Part model, mm, in its own coordinate system. Round coordinates to 2 decimals unless told otherwise and drop trailing zeros. One line per question, with ' | ' between items. Start each with the question number.
1) Drop flat-ended pins along their axis: pin 1 Ø0.5 at (x, y) = (-479, -2) entering from +Z; pin 2 Ø5 at (x, z) = (-476, 6) entering from +Y. Give the stop position or say it passes through.
2) Wall check: probe 1 along Z at (x, y) = (-488, -0.55). Give the ranges that are in metal, low to high. Write a range as [from, to].
3) Mould opens along X. For faces 1 (the face through (-432.766, -2.218, 6.435)), 2 (the face through (-494.696, -2, -1)), 3 (the face through (-445, 0, 0)) say: pulls with the +X half, pulls with the -X half, needs draft (parallel to the pull), parting line crosses it, or undercut.
```python
from build123d import *

# Parameters (mm, degrees)
F1_DEPTH = 4.5


with BuildPart() as f1:
    # F0 (on Front) → F1 (new body)
    with BuildSketch(Plane.XZ):
        Polygon((-494.6955, -7.5), (-394.1515, -7.5), (-394.1515, 5.4), (-394.685, 5.4), (-395.449337, 7.5), (-395.995663, 7.5), (-396.76, 5.4), (-397.827, 5.4), (-398.591337, 7.5), (-399.137663, 7.5), (-399.902, 5.4), (-400.969, 5.4), (-401.733337, 7.5), (-402.279663, 7.5), (-403.044, 5.4), (-404.111, 5.4), (-404.875337, 7.5), (-405.421663, 7.5), (-406.186, 5.4), (-407.253, 5.4), (-408.017337, 7.5), (-408.563663, 7.5), (-409.328, 5.4), (-410.395, 5.4), (-411.159337, 7.5), (-411.705663, 7.5), (-412.47, 5.4), (-413.537, 5.4), (-414.301337, 7.5), (-414.847663, 7.5), (-415.612, 5.4), (-416.679, 5.4), (-417.443337, 7.5), (-417.989663, 7.5), (-418.754, 5.4), (-419.821, 5.4), (-420.585337, 7.5), (-421.131663, 7.5), (-421.896, 5.4), (-422.963, 5.4), (-423.727337, 7.5), (-424.273663, 7.5), (-425.038, 5.4), (-426.105, 5.4), (-426.869337, 7.5), (-427.415663, 7.5), (-428.18, 5.4), (-429.247, 5.4), (-430.011337, 7.5), (-430.557663, 7.5), (-431.322, 5.4), (-432.389, 5.4), (-433.153337, 7.5), (-433.699663, 7.5), (-434.464, 5.4), (-435.531, 5.4), (-436.295337, 7.5), (-436.841663, 7.5), (-437.606, 5.4), (-438.673, 5.4), (-439.437337, 7.5), (-439.983663, 7.5), (-440.748, 5.4), (-441.815, 5.4), (-442.579337, 7.5), (-443.125663, 7.5), (-443.89, 5.4), (-444.957, 5.4), (-445.721337, 7.5), (-446.267663, 7.5), (-447.032, 5.4), (-448.099, 5.4), (-448.863337, 7.5), (-449.409663, 7.5), (-450.174, 5.4), (-451.241, 5.4), (-452.005337, 7.5), (-452.551663, 7.5), (-453.316, 5.4), (-454.383, 5.4), (-455.147337, 7.5), (-455.693663, 7.5), (-456.458, 5.4), (-457.525, 5.4), (-458.289337, 7.5), (-458.835663, 7.5), (-459.6, 5.4), (-460.667, 5.4), (-461.431337, 7.5), (-461.977663, 7.5), (-462.742, 5.4), (-463.809, 5.4), (-464.573337, 7.5), (-465.119663, 7.5), (-465.884, 5.4), (-466.951, 5.4), (-467.715337, 7.5), (-468.261663, 7.5), (-469.026, 5.4), (-470.093, 5.4), (-470.857337, 7.5), (-471.403663, 7.5), (-472.168, 5.4), (-473.235, 5.4), (-473.999337, 7.5), (-474.545663, 7.5), (-475.31, 5.4), (-476.377, 5.4), (-477.141337, 7.5), (-477.687663, 7.5), (-478.452, 5.4), (-479.519, 5.4), (-480.283337, 7.5), (-480.829663, 7.5), (-481.594, 5.4), (-482.661, 5.4), (-483.425337, 7.5), (-483.971663, 7.5), (-484.736, 5.4), (-485.803, 5.4), (-486.567337, 7.5), (-487.113663, 7.5), (-487.878, 5.4), (-488.945, 5.4), (-489.709337, 7.5), (-490.255663, 7.5), (-491.02, 5.4), (-492.087, 5.4), (-492.851337, 7.5), (-493.397663, 7.5), (-494.162, 5.4), (-494.6955, 5.4), align=None)
    extrude(amount=F1_DEPTH)


solid = f1.part
```
Answer key:
1) pin 1: stops at z = 5.4 | pin 2: stops at y = 0
2) probe 1: z = [-7.5, 5.4]
3) face 1: undercut | face 2: pulls with the -X half | face 3: needs draft
